Geometry check sheet. Reference: the model listing, model coordinates, mm. Face numbers are marked on the shaded views. A direction names the side the tool comes from. Round coordinates to 2 decimals unless told otherwise and drop trailing zeros. Write each loop counter-clockwise with the first axis right and the second up, starting at its lowest first coordinate (ties: lowest second). Pieces come first, ordered by that corner, then holes.
from build123d import *

# Parameters (mm, degrees)
F0_W         = 24
F0_H         = 26
F1_DEPTH     = 27
F2_W         = 20
F2_H         = 15.2
F3_DEPTH     = 25
F4_W         = 20
F4_H         = 10
F5_DEPTH     = 24
F7_W         = 3
F7_H         = 14
F8_DEPTH     = 6
F6_W         = 3
F6_H         = 14
F9_DEPTH     = 6
F10_R        = 1.25
F11_DEPTH    = 3
F12_R        = 5
F14_DEPTH    = 48
F15_W        = 3
F15_H        = 30
F16_DEPTH    = 14
F17_T4_DEPTH = 14
F18_R        = 1.65
F19_DEPTH    = 5.8
F21_DEPTH    = 3
F23_DEPTH    = 8.8
F24_DEPTH    = 5
F25_R        = 10
F26_T1_DEPTH = 20
F27_W        = 1
F27_H        = 2
F28_DEPTH    = 3
F29_R        = 5


# Not quite as in the source:
# - a fillet or chamfer that OpenCascade refuses, or shapes differently, is made with other operations: its cross-section is extruded or revolved along the edge and cut away or added


with BuildPart() as f1:
    # F0 (on Top) → F1 (new body)
    with BuildSketch(Plane.XY):
        Rectangle(F0_W, F0_H)
    extrude(amount=F1_DEPTH)

    # F2 (on face) → F3 (cut)
    with BuildSketch(Plane.XY.offset(27)):
        with Locations((0, -3.4)):
            Rectangle(F2_W, F2_H)
    extrude(amount=-F3_DEPTH, mode=Mode.SUBTRACT)

    # F4 (on face) → F5 (cut, through all)
    with BuildSketch(Plane(origin=(0, 13, 0), x_dir=(-1, 0, 0), z_dir=(0, 1, 0))):
        with Locations((0, 7)):
            Rectangle(F4_W, F4_H)
    extrude(amount=-F5_DEPTH, mode=Mode.SUBTRACT)

    # F7 (on face) → F8 (join)
    with BuildSketch(Plane.YZ.offset(12)):
        with Locations((11.5, 7)):
            Rectangle(F7_W, F7_H)
    extrude(amount=F8_DEPTH)

    # F6 (on face) → F9 (join)
    with BuildSketch(Plane(origin=(-12, 0, 0), x_dir=(0, -1, 0), z_dir=(-1, 0, 0))):
        with Locations((-11.5, 7)):
            Rectangle(F6_W, F6_H)
    extrude(amount=F9_DEPTH)

    # F10 (on face) → F11 (cut, through all)
    with BuildSketch(Plane(origin=(0, 13, 0), x_dir=(-1, 0, 0), z_dir=(0, 1, 0))):
        with Locations((-15.5, 7)):
            Circle(F10_R)
        with Locations((15.5, 7)):
            Circle(F10_R)
    extrude(amount=-F11_DEPTH, mode=Mode.SUBTRACT)

    # F12
    f12_edges = [f1.edges().sort_by_distance(p)[0] for p in [
        (18, 11.5, 14),
        (18, 11.5, 0),
        (-18, 11.5, 14),
        (-18, 11.5, 0),
    ]]
    fillet(f12_edges, radius=F12_R)

    # F13 (on face) → F14 (join)
    with BuildSketch(Plane.XY.offset(27)):
        Polygon((2, 13), (-12, 13), (-12, 4.2), (-10, 4.2), (2, 4.2), align=None)
    extrude(amount=F14_DEPTH)

    # F15 (on face) → F16 (cut, through all)
    with BuildSketch(Plane(origin=(-12, 0, 0), x_dir=(0, -1, 0), z_dir=(-1, 0, 0))):
        with Locations((-11.5, 60)):
            Rectangle(F15_W, F15_H)
    extrude(amount=-F16_DEPTH, mode=Mode.SUBTRACT)

    # F17: chamfer of 3 x 4 on 1 edges, made by hand


with BuildPart() as f17_tool2:
    # F17_s3 → F17_t4 (new body)
    with BuildSketch(Plane.YZ.offset(-12)):
        Polygon((14, 45), (10, 48), (10, 45), align=None)
    extrude(amount=F17_T4_DEPTH)

    split(bisect_by=Plane.XZ.offset(-13), keep=Keep.TOP)


with BuildPart() as f1_1:
    add(f1.part)

    # F17_t1: union F17_tool2
    add(f17_tool2.part)

    # F18 (on face) → F19 (cut, through all)
    with BuildSketch(Plane.XZ.offset(-4.2)):
        with Locations((-5, 70)):
            Circle(F18_R)
    extrude(amount=-F19_DEPTH, mode=Mode.SUBTRACT)

    # F20 (on face) → F21 (cut)
    with BuildSketch(Plane(origin=(0, 10, 0), x_dir=(-1, 0, 0), z_dir=(0, 1, 0))):
        Polygon((8.4994896827, 70.0597658786), (6.6979860722, 73.0605299049), (3.1984963894, 73.0007640263), (1.5005103171, 69.9402341215), (3.3020139276, 66.9394700952), (6.8015036104, 66.9992359738), align=None)
    extrude(amount=-F21_DEPTH, mode=Mode.SUBTRACT)

    # F22 (on face) → F23 (cut, through all)
    with BuildSketch(Plane(origin=(0, 13, 0), x_dir=(-1, 0, 0), z_dir=(0, 1, 0))):
        with BuildLine():
            ThreePointArc((3.1, 22.625), (0, 25.725), (-3.1, 22.625))
            Line((-3.1, 22.625), (-3.1, 16.725))
            ThreePointArc((-3.1, 16.725), (0, 13.625), (3.1, 16.725))
            Line((3.1, 16.725), (3.1, 22.625))
        make_face()
        with BuildLine():
            Line((1.7, 20.925), (1.7, 18.425))
            ThreePointArc((1.7, 18.425), (1.202081528, 17.222918472), (0, 16.725))
            ThreePointArc((0, 16.725), (-1.202081528, 17.222918472), (-1.7, 18.425))
            Line((-1.7, 18.425), (-1.7, 20.925))
            ThreePointArc((-1.7, 20.925), (-1.202081528, 22.127081528), (0, 22.625))
            ThreePointArc((0, 22.625), (1.202081528, 22.127081528), (1.7, 20.925))
        make_face(mode=Mode.SUBTRACT)
        with BuildLine():
            ThreePointArc((9.1, 41.95), (6, 45.05), (2.9, 41.95))
            Line((2.9, 41.95), (2.9, 36.05))
            ThreePointArc((2.9, 36.05), (6, 32.95), (9.1, 36.05))
            Line((9.1, 36.05), (9.1, 41.95))
        make_face()
        with BuildLine():
            ThreePointArc((4.3, 40.25), (4.797918472, 41.452081528), (6, 41.95))
            ThreePointArc((6, 41.95), (7.202081528, 41.452081528), (7.7, 40.25))
            Line((7.7, 40.25), (7.7, 37.75))
            ThreePointArc((7.7, 37.75), (7.202081528, 36.547918472), (6, 36.05))
            ThreePointArc((6, 36.05), (4.797918472, 36.547918472), (4.3, 37.75))
            Line((4.3, 37.75), (4.3, 40.25))
        make_face(mode=Mode.SUBTRACT)
        with BuildLine():
            ThreePointArc((-1.7, 18.425), (-1.202081528, 17.222918472), (0, 16.725))
            Line((0, 16.725), (0, 22.625))
            ThreePointArc((0, 22.625), (-1.202081528, 22.127081528), (-1.7, 20.925))
            Line((-1.7, 20.925), (-1.7, 18.425))
        make_face()
        with BuildLine():
            ThreePointArc((0, 16.725), (1.202081528, 17.222918472), (1.7, 18.425))
            Line((1.7, 18.425), (1.7, 20.925))
            ThreePointArc((1.7, 20.925), (1.202081528, 22.127081528), (0, 22.625))
            Line((0, 22.625), (0, 16.725))
        make_face()
        with BuildLine():
            Line((6, 41.95), (6, 40.25))
            Line((6, 40.25), (6, 37.75))
            Line((6, 37.75), (6, 36.05))
            ThreePointArc((6, 36.05), (7.202081528, 36.547918472), (7.7, 37.75))
            Line((7.7, 37.75), (7.7, 40.25))
            ThreePointArc((7.7, 40.25), (7.202081528, 41.452081528), (6, 41.95))
        make_face()
        with BuildLine():
            Line((6, 37.75), (6, 40.25))
            Line((6, 40.25), (6, 41.95))
            ThreePointArc((6, 41.95), (4.797918472, 41.452081528), (4.3, 40.25))
            Line((4.3, 40.25), (4.3, 37.75))
            ThreePointArc((4.3, 37.75), (4.797918472, 36.547918472), (6, 36.05))
            Line((6, 36.05), (6, 37.75))
        make_face()
    extrude(amount=-F23_DEPTH, mode=Mode.SUBTRACT)

    # F22 (on face) → F24 (join)
    with BuildSketch(Plane(origin=(0, 13, 0), x_dir=(-1, 0, 0), z_dir=(0, 1, 0))):
        with BuildLine():
            ThreePointArc((3.1, 22.625), (0, 25.725), (-3.1, 22.625))
            Line((-3.1, 22.625), (-3.1, 16.725))
            ThreePointArc((-3.1, 16.725), (0, 13.625), (3.1, 16.725))
            Line((3.1, 16.725), (3.1, 22.625))
        make_face()
        with BuildLine():
            Line((1.7, 20.925), (1.7, 18.425))
            ThreePointArc((1.7, 18.425), (1.202081528, 17.222918472), (0, 16.725))
            ThreePointArc((0, 16.725), (-1.202081528, 17.222918472), (-1.7, 18.425))
            Line((-1.7, 18.425), (-1.7, 20.925))
            ThreePointArc((-1.7, 20.925), (-1.202081528, 22.127081528), (0, 22.625))
            ThreePointArc((0, 22.625), (1.202081528, 22.127081528), (1.7, 20.925))
        make_face(mode=Mode.SUBTRACT)
        with BuildLine():
            ThreePointArc((9.1, 41.95), (6, 45.05), (2.9, 41.95))
            Line((2.9, 41.95), (2.9, 36.05))
            ThreePointArc((2.9, 36.05), (6, 32.95), (9.1, 36.05))
            Line((9.1, 36.05), (9.1, 41.95))
        make_face()
        with BuildLine():
            ThreePointArc((4.3, 40.25), (4.797918472, 41.452081528), (6, 41.95))
            ThreePointArc((6, 41.95), (7.202081528, 41.452081528), (7.7, 40.25))
            Line((7.7, 40.25), (7.7, 37.75))
            ThreePointArc((7.7, 37.75), (7.202081528, 36.547918472), (6, 36.05))
            ThreePointArc((6, 36.05), (4.797918472, 36.547918472), (4.3, 37.75))
            Line((4.3, 37.75), (4.3, 40.25))
        make_face(mode=Mode.SUBTRACT)
    extrude(amount=-F24_DEPTH)

    # F25
    f25_edges = [f1_1.edges().sort_by_distance(p)[0] for p in [
        (0, -13, 0),
        (0, -11, 2),
    ]]
    fillet(f25_edges, radius=F25_R)

    # F26: fillet of radius 5 on 1 edges, made by hand

    # F26_s2 → F26_t1 (cut)
    with BuildSketch(Plane.YZ.offset(-10)):
        with BuildLine():
            ThreePointArc((4.2, 17), (5.6644660941, 13.4644660941), (9.2, 12))
            Line((9.2, 12), (4.2, 12))
            Line((4.2, 12), (4.2, 17))
        make_face()
    extrude(amount=F26_T1_DEPTH, mode=Mode.SUBTRACT)

    # F27 (on face) → F28 (cut)
    with BuildSketch(Plane.XY.offset(27)):
        with Locations((-10.5, -3.3)):
            Rectangle(F27_W, F27_H)
    extrude(amount=-F28_DEPTH, mode=Mode.SUBTRACT)

    # F29
    f29_edges = [f1_1.edges().sort_by_distance(p)[0] for p in [
        (-12, 7.1, 75),
        (2, 7.1, 75),
    ]]
    fillet(f29_edges, radius=F29_R)


solid = f1_1.part
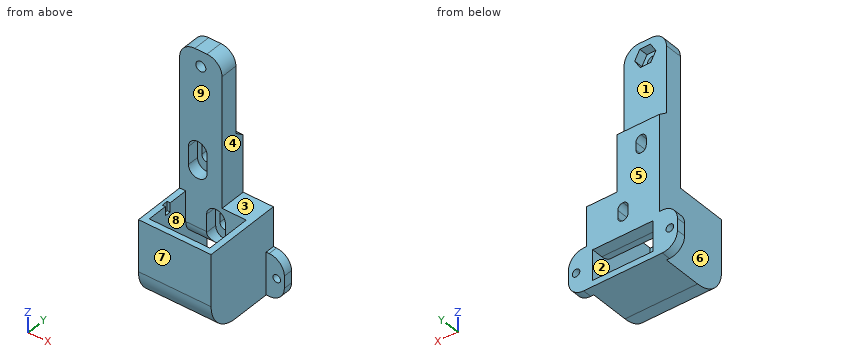
1. Section check B-B (y = 0.5). Record the cut outline in (x, z).
2. Section check D-D (z = 63.5). Record the cut outline in (x, y).
3. Depth check by flat-ended pin: pin 1 Ø1.2 at (y, z) = (10, 39.5) entering from +X; pin 2 Ø5 at (x, z) = (-4, 68.5) entering from +Y; pin 3 Ø1.8 at (x, z) = (-14, 5.5) entering from -Y; pin 4 Ø2 at (x, z) = (-15.5, 7) entering from -Y. Enter the tip coordinate at first touch or a pass-through.
4. Access from +Z, -Z, +X, -X, +Y, -Y to the whole of each face (thin tool, end or side, straight path). Record for the marked faces 1, 2, 3, 4 and 5.
5. Section check C-C (x = -5). State how many separate pieces and enclosed holes the cut face has, plus the area to 3 significant figures.
6. Scan lines: line 1 along X through (y, z) = (-7, 23.5); line 2 along X through (y, z) = (6.1, 70); line 3 along Z through (x, y) = (-5, 9.75). Record each from-to range of solid material in increasing order.
7. Release check for a two-part mould opening along Y. For the marked faces 6, 7, 8 and 9 record: +Y half, -Y half, draft (parallel to the pull), parting line (faces both ways), or undercut.
8. Section check A-A (x = -15.5). Record the cut outline in (y, z).
Results below:
1. outline: (-12, 0) - (12, 0) - (12, 27) - (10, 27) - (10, 2) - (-10, 2) - (-10, 27) - (-12, 27) - close
2. outline: (-12, 4.2) - (2, 4.2) - (2, 10) - (-12, 10) - close
3. pin 1: stops at x = 2
3. pin 2: stops at y = 10
3. pin 3: stops at y = 10
3. pin 4: passes through
4. face 1: +Z, +X, -X, +Y
4. face 2: none
4. face 3: +Z, +X, -Y
4. face 4: +Z, +X, +Y, -Y
4. face 5: +Z, -Z, +X, -X, +Y
5. separate pieces: 4
5. enclosed holes: 0
5. area: 468 mm2
6. line 1: x = -12 to -10, 10 to 12
6. line 2: x = -12 to -6.65, -3.35 to 2
6. line 3: z = 0 to 2, 12 to 36.38, 41.62 to 66.97, 73.03 to 75
7. face 6: draft
7. face 7: -Y half
7. face 8: undercut
7. face 9: undercut
8. outline: (10, 0.67) - (13, 0.67) - (13, 5.75) - (10, 5.75) - close; (10, 8.25) - (13, 8.25) - (13, 13.33) - (10, 13.33) - close
